Geometry: see drawing. Coordinates: mm, zero at the bounding-box minimum. A direction names the side the tool comes from. Coordinates: 2 decimals unless noted, no trailing zeros. Write each loop counter-clockwise with the first axis right and the second up, starting at its lowest first coordinate (ties: lowest second). Pieces come first, ordered by that corner, then holes. Notation, with made-up numbers: (-13.75, 74.5) -> (-8.75, 74.5) arc R11 ccw to (-8.75, 88.5) -> close; hole circle Ø4 at (-12, 39). An arc over 180 degrees is marked (long way). Use one line per item in the form item = value. Start each with the question number.
(1) Pull-direction query (Y, two-part tool) for the marked faces 3, 4 and 5; classes: released by +Y, released by -Y, zero draft, split by the parting line, or undercut.
(2) First-contact query: pin 1 (2 mm diameter, centred on x = 22, z = 0.5, fed in from -Y); pin 2 (15.5 mm diameter, centred on y = 6, z = 21, fed in from -X); pin 3 (2 mm diameter, centred on x = 41.5, z = 34, fed in from -Y). Flat tips, straight axial feed; report the tip coordinate or a pass-through.
(3) Ray query, line 1 along Z through (x, y) = (9.5, 23); line 2 along Z through (x, y) = (24.5, 34); line 3 along Y through (x, z) = (3, 29.5). Return the intervals inside material, ascending.
(4) Cut plane B-B on x = 28. Return the cut outline in (y, z).
(5) Cut plane C-C on z = 12. Return the cut outline in (x, y), plus the area to 3 significant figures.
(6) Cut plane A-A on y = 17. Return the cut outline in (x, z), plus the area to 3 significant figures.
(7) Set-up query: the marked faces 1 and 2. Return all of +Z, -Z, +X, -X, +Y, -Y with unobstructed straight access to the full face (end or side cutting, diameter ignored); none if empty.
(8) Cut plane D-D on x = 39. Return the cut outline in (y, z), plus the area to 3 significant figures.
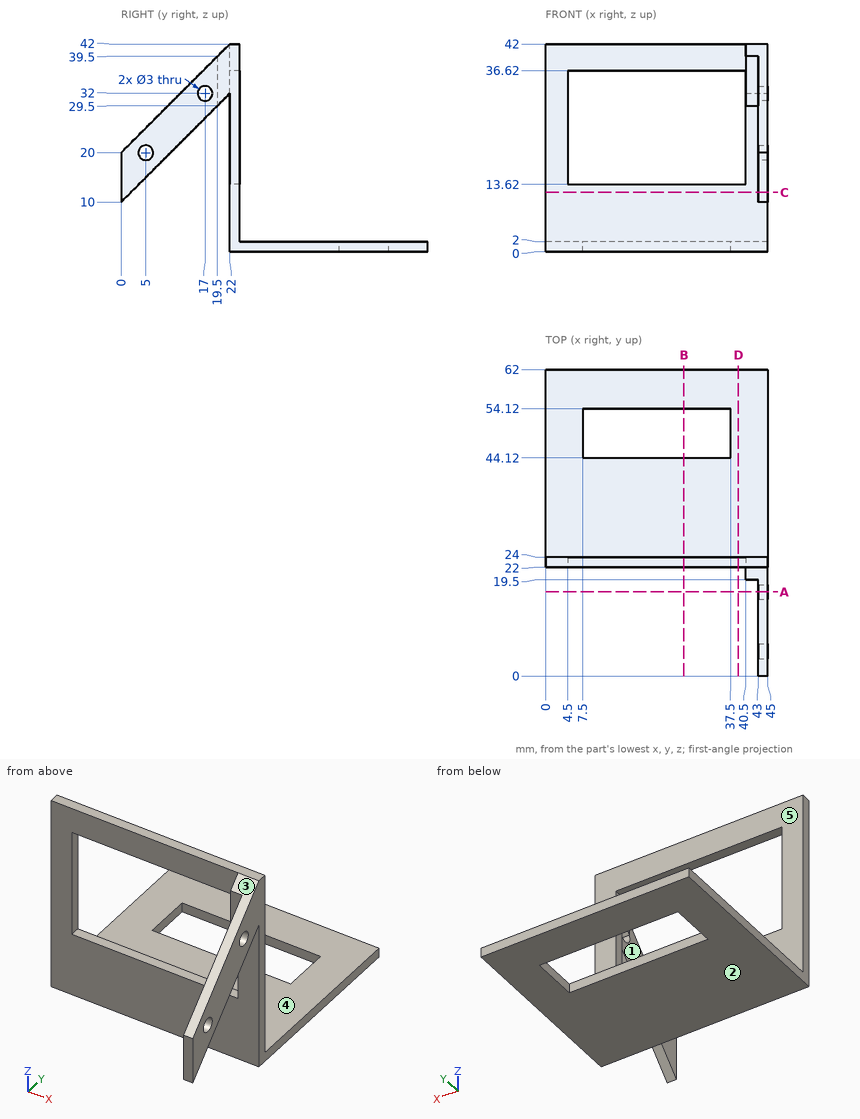
Values:
q1.face_3 = released by -Y
q1.face_4 = zero draft
q1.face_5 = released by +Y
q2.pin_1 = 22
q2.pin_2 = 43
q2.pin_3 = 19.5
q3.line_1 = 0 to 13.62, 36.62 to 42
q3.line_2 = 0 to 2
q3.line_3 = 22 to 24
q4.outline = (22, 0) -> (44.12, 0) -> (44.12, 2) -> (24, 2) -> (24, 13.62) -> (22, 13.62) -> close; (22, 36.62) -> (24, 36.62) -> (24, 42) -> (22, 42) -> close; (54.12, 0) -> (62, 0) -> (62, 2) -> (54.12, 2) -> close
q5.outline = (0, 22) -> (45, 22) -> (45, 24) -> (0, 24) -> close; (43, 0) -> (45, 0) -> (45, 2) -> (43, 2) -> close
q5.area = 94.0 mm2
q6.outline = (43, 27) -> (45, 27) -> (45, 30.5) -> (43, 30.5) -> close; (43, 33.5) -> (45, 33.5) -> (45, 37) -> (43, 37) -> close
q6.area = 14.0 mm2
q7.face_1 = +Z, -Z, -X, -Y
q7.face_2 = -Z, +X, -X, +Y, -Y
q8.outline = (22, 0) -> (62, 0) -> (62, 2) -> (24, 2) -> (24, 13.62) -> (22, 13.62) -> close; (22, 36.62) -> (24, 36.62) -> (24, 42) -> (22, 42) -> close
q8.area = 114 mm2
